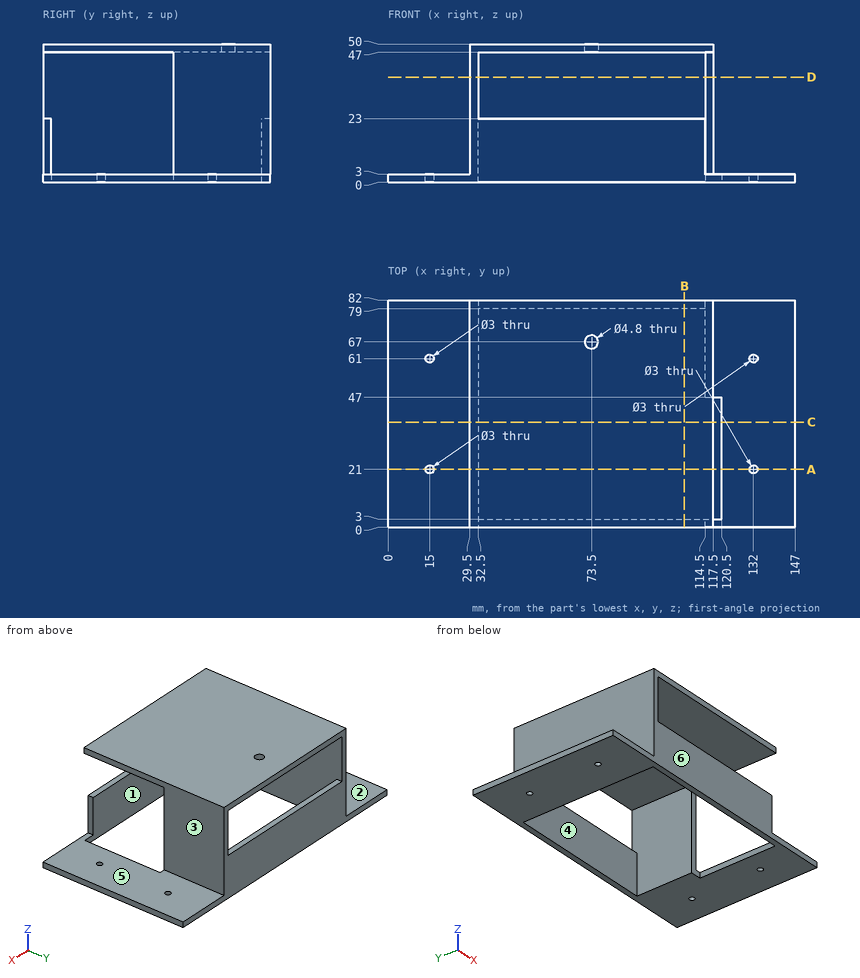
Geometry check sheet. Reference: drawing and pictorial views, mm from the part's lowest x, y, z. A direction names the side the tool comes from. Give positions to 0.01 mm unless a question says otherwise; leave off trailing zeros. Write each loop counter-clockwise with the first axis right and the second up, starting at its lowest first coordinate (ties: lowest second). Pieces come first, ordered by that corner, then holes. Notation, with made-up numbers: (50.5, 55) - (102.5, 55) arc R29 ccw to (102.5, 76) - close; hole circle Ø11 at (-1, 80.5). An arc over 180 degrees is marked (long way). Put each result on its own line as item: value.
Q1. Depth check by flat-ended pin: P1, Ø2.5, axis at y = 1.5, z = 14, coming from the +X side; P2, Ø1.5, axis at y = 50.5, z = 21, coming from the -X side; P3, Ø14, axis at y = 36, z = 16, coming from the +X side; P4, Ø1.8, axis at x = 15, y = 21, coming from the +Z side. Enter the tip coordinate at first touch or a pass-through.
Result:
P1: x = 114.5
P2: x = 29.5
P3: x = 32.5
P4: through
Q2. Scan lines: probe 1 along Y at (x, z) = (132, 1); probe 2 along Y at (x, z) = (72, 12); probe 3 along X at (y, z) = (53, 39.5). Record each from-to range of solid material in increasing order. Write a range as from..to.
Result:
probe 1: 0..19.5, 22.5..59.5, 62.5..82
probe 2: 0..3, 79..82
probe 3: 29.5..32.5, 114.5..117.5
Q3. Section check C-C on y = 38. Record the cut outline in (x, z), and give its area (3 significant figures).
Result:
outline: (0, 0) - (32.5, 0) - (32.5, 47) - (117.5, 47) - (117.5, 50) - (29.5, 50) - (29.5, 3) - (0, 3) - close; (120.5, 0) - (147, 0) - (147, 3) - (120.5, 3) - close
area: 573 mm2
Q4. Section check D-D on z = 38. Record the cut outline in (x, y), and give its area (3 significant figures).
Result:
outline: (29.5, 0) - (32.5, 0) - (32.5, 82) - (29.5, 82) - close; (114.5, 47) - (117.5, 47) - (117.5, 82) - (114.5, 82) - close
area: 351 mm2
Q5. Section check A-A on y = 21. Record the cut outline in (x, z).
Result:
outline: (0, 0) - (13.5, 0) - (13.5, 3) - (0, 3) - close; (16.5, 0) - (32.5, 0) - (32.5, 47) - (117.5, 47) - (117.5, 50) - (29.5, 50) - (29.5, 3) - (16.5, 3) - close; (120.5, 0) - (130.5, 0) - (130.5, 3) - (120.5, 3) - close; (133.5, 0) - (147, 0) - (147, 3) - (133.5, 3) - close
Q6. Section check B-B on x = 107. Record the cut outline in (y, z).
Result:
outline: (0, 0) - (3, 0) - (3, 23) - (0, 23) - close; (0, 47) - (82, 47) - (82, 50) - (0, 50) - close; (79, 0) - (82, 0) - (82, 23) - (79, 23) - close
Q7. Mould release check, pull along Y, two halves, no side actions. Record for the marked faces 4, 5 and 6: released by +Y, released by -Y, zero draft, split by the parting line, or undercut.
Result:
face 4: undercut
face 5: zero draft
face 6: released by -Y
Q8. Set-up check for the marked faces 1, 2 and 3: record each of +Z, -Z, +X, -X, +Y, -Y from which the full face is reachable in a straight line by a thin tool's end or side.
Result:
face 1: -Z
face 2: +Z, -X, +Y, -Y
face 3: +Z, +X, +Y, -Y
